```python
from build123d import *

# Parameters (mm, degrees)
SKETCH1_R          = 23.6855
EXTRUDE1_DEPTH     = 66.548
CHAMFER1_SIZE      = 0.762
SKETCH6_R          = 17.4625
EXTRUDE2_DEPTH     = 5.969
SKETCH7_W          = 20.828
SKETCH7_H          = 10.31875
CUT_EXTRUDE4_DEPTH = 19.84248
HOLE1_D            = 4.7498
HOLE1_DEPTH        = 4.7498
CIRPATTERN1_COUNT  = 4
LPATTERN1_COUNT    = 2
LPATTERN1_PITCH    = 28.5496


with BuildPart() as part:
    # Sketch1 → Extrude1 (new body)
    with BuildSketch(Plane.XY):
        Circle(SKETCH1_R)
    extrude(amount=EXTRUDE1_DEPTH)

    # Sketch2 → Cut-Revolve1 (revolve, cut)
    with BuildSketch(Plane(origin=(0, 0, 0), x_dir=(1, 0, 0), z_dir=(0, 1, 0)), mode=Mode.PRIVATE) as cut_revolve1_sk:
        Polygon((23.6855, -66.548), (23.6855, -52.578), (22.4155, -53.848), (22.4155, -66.548), align=None)
    revolve(cut_revolve1_sk.sketch.rotate(Axis((0, 0, 0), (0, 0, 1)), 180), axis=Axis((0, 0, 0), (0, 0, 1)), mode=Mode.SUBTRACT)  # turned: the seam where the file's is

    # Sketch3 → Cut-Revolve2 (revolve, cut)
    with BuildSketch(Plane(origin=(0, 0, 0), x_dir=(1, 0, 0), z_dir=(0, 1, 0)), mode=Mode.PRIVATE) as cut_revolve2_sk:
        Polygon((22.4155, 0), (22.4155, -1.524), (23.6855, -2.794), (23.6855, 0), align=None)
    revolve(cut_revolve2_sk.sketch.rotate(Axis((0, 0, 0), (0, 0, -1)), 180), axis=Axis((0, 0, 0), (0, 0, -1)), mode=Mode.SUBTRACT)  # turned: the seam where the file's is

    # Chamfer1
    chamfer1_edges = [part.edges().sort_by_distance(p)[0] for p in [
        (22.4155, 0, 66.548),
    ]]
    chamfer(chamfer1_edges, length=CHAMFER1_SIZE)

    # S2D0002 → Cut-Revolve3 (revolve, cut)
    with BuildSketch(Plane(origin=(0, 0, 0), x_dir=(0, -1, 0), z_dir=(1, 0, 0)), mode=Mode.PRIVATE) as cut_revolve3_sk:
        Polygon((20.4597, -66.294), (23.7998, -66.294), (23.7998, -66.548), (14.2748, -66.548), (14.2748, -52.324), (19.2532, -52.324), (19.2532, -63.077393135), (19.917106865, -63.7413), align=None)
    cut_revolve3 = revolve(cut_revolve3_sk.sketch.rotate(Axis((0, -14.2748, 14.6685), (0, 0, -1)), 270), axis=Axis((0, -14.2748, 14.6685), (0, 0, -1)), mode=Mode.SUBTRACT)  # turned: the seam where the file's is

    # Sketch6 → Extrude2 (add)
    with BuildSketch(Plane(origin=(0, 0, 0), x_dir=(-1, 0, 0), z_dir=(0, 0, -1))):
        with Locations(Location((0, 0, 0), (0, 0, 180))):  # turned: the seam where the file's is
            Circle(SKETCH6_R)
    extrude(amount=EXTRUDE2_DEPTH)

    # Sketch7 → Revolve1 (revolve)
    with BuildSketch(Plane(origin=(0, 0, 0), x_dir=(0, 0, -1), z_dir=(1, 0, 0)), mode=Mode.PRIVATE) as revolve1_sk:
        with Locations((16.383, -5.159375)):
            Rectangle(SKETCH7_W, SKETCH7_H)
    revolve(revolve1_sk.sketch.rotate(Axis((0, 0, 0), (0, 0, -1)), 90), axis=Axis((0, 0, 0), (0, 0, -1)))  # turned: the seam where the file's is

    # S2D0001 → Cut-Revolve5 (revolve, cut)
    with BuildSketch(Plane(origin=(0, 0, 0), x_dir=(1, 0, 0), z_dir=(0, 1, 0))):
        Polygon((3.2639, 24.861260017), (3.2639, 11.9888), (0, 11.9888), (0, 26.797), (4.3815, 26.797), align=None)
    revolve(axis=Axis((0, 0, 31.308359971), (0, 0, -1)), mode=Mode.SUBTRACT)

    # Sketch9 → Cut-Revolve6 (revolve, cut)
    with BuildSketch(Plane(origin=(0, 0, 0), x_dir=(0, -1, 0), z_dir=(1, 0, 0)), mode=Mode.PRIVATE) as cut_revolve6_sk:
        with BuildLine():
            Line((-10.31875, 19.3802), (-10.033, 20.1422))
            Line((-10.033, 20.1422), (-10.033, 25.781))
            ThreePointArc((-10.033, 25.781), (-9.932678675, 26.324796865), (-9.644922533, 26.797))
            Line((-9.644922533, 26.797), (-10.31875, 26.797))
            Line((-10.31875, 26.797), (-10.31875, 19.3802))
        make_face()
    revolve(cut_revolve6_sk.sketch.rotate(Axis((0, 0, -12.65936), (0, 0, -1)), 90), axis=Axis((0, 0, -12.65936), (0, 0, -1)), mode=Mode.SUBTRACT)  # turned: the seam where the file's is

    # Sketch13 → Cut-Extrude4 (cut, symmetric)
    with BuildSketch(Plane(origin=(0, 0, 0), x_dir=(1, 0, 0), z_dir=(0, 1, 0))):
        Polygon((8.5852, 26.797), (8.5852, 21.844), (10.033, 20.3962), (10.033, 26.797), align=None)
        Polygon((-8.5852, 26.797), (-8.5852, 21.844), (-10.033, 20.3962), (-10.033, 26.797), align=None)
    extrude(amount=CUT_EXTRUDE4_DEPTH, both=True, mode=Mode.SUBTRACT)

    # Hole1
    with Locations(Plane(origin=(-15.850152054, 15.850152054, 60.198), x_dir=(0.707106781, 0.707106781, 0), z_dir=(-0.707106781, 0.707106781, 0))):
        with Locations((0, 0)):
            hole1 = Hole(HOLE1_D / 2, depth=HOLE1_DEPTH)

    # CirPattern1: Hole1 ×4 about axis
    cirpattern1_axis = Axis((0, 0, 0), (0, 0, 1))
    for i in range(1, CIRPATTERN1_COUNT):
        add(hole1.rotate(cirpattern1_axis, i * 360 / CIRPATTERN1_COUNT), mode=Mode.SUBTRACT)

    # LPattern1: Cut-Revolve3 ×2
    with Locations(*[(0, i * LPATTERN1_PITCH, 0) for i in range(1, LPATTERN1_COUNT)]):
        add(cut_revolve3, mode=Mode.SUBTRACT)


solid = part.part
```
For this review, take the finished solid that the model builds, in its own axes (mm). A direction names the side the tool comes from. Coordinates: 2 decimals unless noted, no trailing zeros. Loops run counter-clockwise (first coordinate to the right, second up) from the corner with the lowest first, then second, coordinate; pieces in that order, holes last.
1. Mouldability with a two-part tool opening along Y and no side actions: class faces 5 (the conical face through (-20.11, 8.34, 66.43)), 6 (the flat face through (-8.585, 0, -24)), 7 (the flat face through (12.515, 12.468, 60.165)) as +Y half, -Y half, draft (parallel to the pull), parting line (faces both ways), or undercut.
2. For faces 1 (the flat face through (3.94, 2.28, -26.797)), 2 (the flat face through (0, 0, -11.989)), 3 (the flat face through (0.1, -7.7, 66.294)), 4 (the flat face through (-12.515, -12.468, 60.165)), list the 3-axis set-ups (+Z, -Z, +X, -X, +Y, -Y) from which the entire face can be reached by the end or side of a thin tool; tool diameter is ignored.
3. Insertion check: P1, Ø6, axis at x = 0, y = 14.27, coming from the -Z side; P2, Ø5.5, axis at y = -1, z = -24.5, coming from the -X side; P3, Ø12, axis at y = -12, z = -3, coming from the -X side. Each pin has a flat end and moves straight along its axis. Give the tip position at first contact, or say it passes through.
4. Add section C-C, the plane z = 10.5. Give the boundary of the cut face in (x, y), then the cut area to 3 significant figures.
5. Add section B-B, the plane x = -13. Count the separate pieces of the cut face and the enclosed holes in it, then the cut area to 3 significant figures.
6. Add section A-A, the plane z = -8.5. Give the boundary of the cut face in (x, y).
7. For line 1 (Y direction, x = 0, z = 56.25); line 2 (Y direction, x = 0, z = -17); line 3 (Y direction, x = 0, z = 66), list the stretches that pass through material, from the lowest coordinate up.
Result:
1. face 5: parting line
1. face 6: draft
1. face 7: undercut
2. face 1: -Z, +X, -X, +Y, -Y
2. face 2: -Z
2. face 3: +Z
2. face 4: none
3. P1: stops at z = -5.97
3. P2: stops at x = -8.68
3. P3: stops at x = -21.36
4. outline: circle Ø47.37 at (0, 0)
4. area: 1,760 mm2
5. separate pieces: 1
5. enclosed holes: 2
5. area: 2,690 mm2
6. outline: circle Ø20.64 at (0, 0)
7. line 1: y = -22.42 to -19.25, -9.3 to 9.3, 19.25 to 22.42
7. line 2: y = -10.32 to -3.26, 3.26 to 10.32
7. line 3: y = -22.2 to -20.4, -8.15 to 8.15, 20.4 to 22.2
